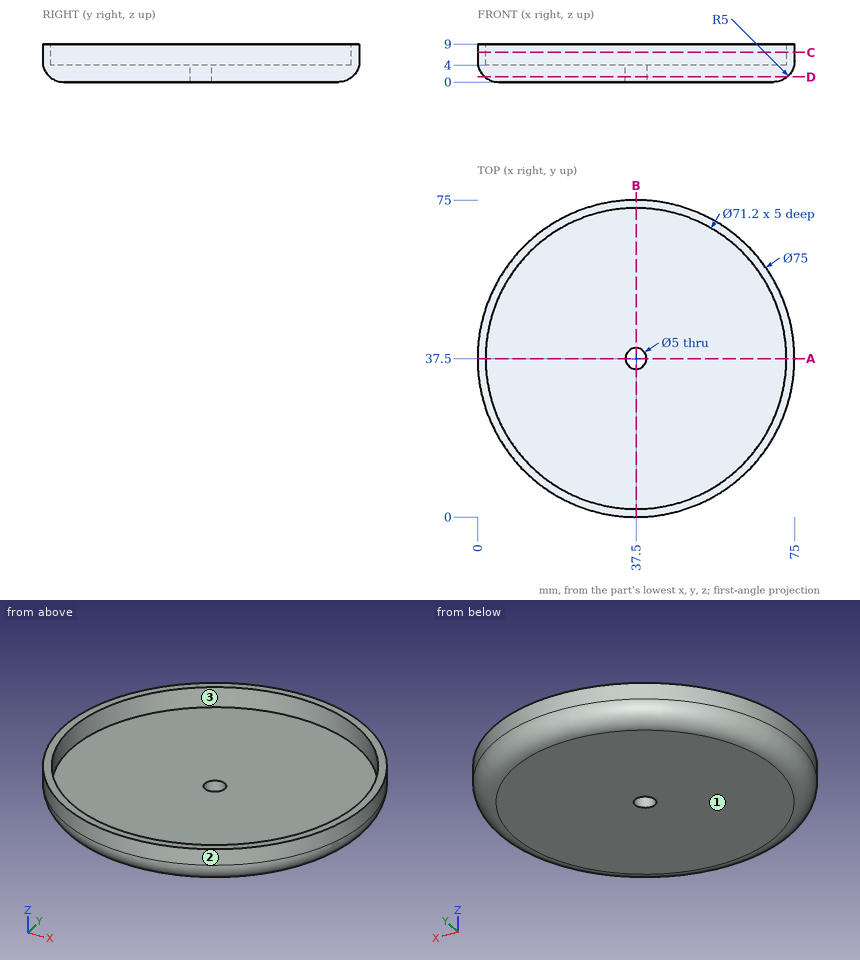
For this review, use the dimensioned drawing (mm, ordinates from the lowest corner) and the shaded views. Round coordinates to 2 decimals unless told otherwise and drop trailing zeros. Order: outer loops, then holes, each group sorted by start corner. A loop starts at its lowest first (then second) coordinate and runs counter-clockwise, first axis right, second up. Notation, with made-up numbers: M -39,45.5 L -5,45.5 A32 cw -5,77.5 Z; hole C -33,-6.75 d7. An arc over 180 degrees is marked long. Use a Markdown table: item, result.
1) Consider section A-A (y = 37.5). Write out the cut boundary in (x, z), then the cut area to 3 significant figures.
Report:
| item | result |
|---|---|
| outline | M 0,5 A5 ccw 5,0 L 35,0 L 35,4 L 1.9,4 L 1.9,9 L 0,9 Z; M 40,0 L 70,0 A5 ccw 75,5 L 75,9 L 73.1,9 L 73.1,4 L 40,4 Z |
| area | 288 mm^2 |
2) Insertion check: pin 1 (2 mm diameter, centred on y = 35, z = 4.5, fed in from +X); pin 2 (3 mm diameter, centred on x = 40.5, z = 3.5, fed in from -Y); pin 3 (6.5 mm diameter, centred on x = 37.5, y = 37.5, fed in from +Z); pin 4 (12 mm diameter, centred on x = 15, y = 34, fed in from -Z). Each pin has a flat end and moves straight along its axis. Give the tip position at first contact, or say it passes through.
Report:
| item | result |
|---|---|
| pin 1 | x = 74.97 |
| pin 2 | y = 0.07 |
| pin 3 | z = 4 |
| pin 4 | z = 0 |
3) Draft analysis for pull direction Y (two halves, no side actions). For the marked faces 1, 2 and 3, state which applies: released by +Y, released by -Y, zero draft, split by the parting line, or undercut.
Report:
| item | result |
|---|---|
| face 1 | zero draft |
| face 2 | split by the parting line |
| face 3 | undercut |
4) Consider section D-D (z = 1.25). Write out the cut boundary in (x, y), then the cut area to 3 significant figures.
Report:
| item | result |
|---|---|
| outline | C 37.5,37.5 d71.61; hole C 37.5,37.5 d5 |
| area | 4,010 mm^2 |
5) Wall thickness on line 1 along Y through (x, z) = (37.5, 7); line 2 along Z through (x, y) = (13, 48); line 3 along X through (y, z) = (39.5, 7): over which ranges is each line inside the solid? List them lowest first. Write a range as [from, to].
Report:
| item | result |
|---|---|
| line 1 | [0, 1.9], [73.1, 75] |
| line 2 | [0, 4] |
| line 3 | [0.05, 1.96], [73.04, 74.95] |
6) Consider section C-C (z = 7). Write out the cut boundary in (x, y), then the cut area to 3 significant figures.
Report:
| item | result |
|---|---|
| outline | C 37.5,37.5 d75; hole C 37.5,37.5 d71.2 |
| area | 436 mm^2 |
